The listing builds one solid part. Answer for the finished solid, in the listing's coordinates (mm). A direction names the side the tool comes from. Give positions to 0.01 mm unless a question says otherwise; leave off trailing zeros. Order: outer loops, then holes, each group sorted by start corner. A loop starts at its lowest first (then second) coordinate and runs counter-clockwise, first axis right, second up. Notation, with made-up numbers: (64, 59.25) - (120, 59.25) arc R15 ccw to (120, 77.25) - close; hole circle Ø11 at (34, -11). An arc over 180 degrees is marked (long way). Answer as CSV lines item,"result". Start each with the question number.
1. Section B-B on y = 21.5 is taken. Give the vertices of the cut face in (x, z) (3 decimals), and give its area (3 significant figures).
2. Section A-A on x = -26 is taken. Give the vertices of the cut face in (y, z) (3 decimals).
3. Consider line 1 along X through (y, z) = (4, 0.5); line 2 along X through (y, z) = (1.5, 2.75); line 3 along X through (y, z) = (22, 2.3). Determine where each line is inside the solid, lowest interval first. Write a range as [from, to].
4. Determine the mould class of faces 6 (the flat face through (-47, 79.301, 2)), 7 (the flat face through (-32.899, 4, 2)), 8 (the flat face through (-2, -3.884, 2)), 9 (the flat face through (50.286, 22, 2)) for opening direction X: +X half, -X half, draft (parallel to the pull), parting line (faces both ways), or undercut.
5. Which of the six approach directions +Z, -Z, +X, -X, +Y, -Y give full straight-line access (tool end or side, diameter ignored) to faces 1 (the flat face through (-32.899, -2, 2)), 2 (the flat face through (-1.307, 2, 2)), 3 (the flat face through (52, 26.926, 2)), 4 (the flat face through (-47, 1.831, 2)), 5 (the flat face through (-47, 45.493, 2))?
6. Flat-ended cylindrical pins translate along their axes: pin 1 (1 mm diameter, centred on x = -46, z = 1.5, fed in from -Y); pin 2 (1 mm diameter, centred on y = 44, z = 1, fed in from -X); pin 3 (1 mm diameter, centred on y = -6, z = 1, fed in from +X). Find the tip coordinate at first contact, or state that the pin passes through.
from build123d import *

# Parameters (mm, degrees)
F0_W     = 3.175
F0_H     = 6.35
F0_W_2   = 3.5052
F0_H_2   = 4.445
F0_H_3   = 2.778125
F0_W_3   = 2.21615
F0_H_4   = 2.301875
F1_DEPTH = 3.175


with BuildPart() as f1:
    # F0 (on Top) → F1 (new body)
    with BuildSketch(Plane.XY):
        with BuildLine():
            Line((-39.248683933, 94.5405161858), (-44.963683933, 94.5405161858))
            Line((-44.963683933, 94.5405161858), (-44.963683933, 85.6505161858))
            Line((-44.963683933, 85.6505161858), (-44.963683933, 79.3005161858))
            Line((-44.963683933, 79.3005161858), (-44.963683933, 75.7953161858))
            Line((-44.963683933, 75.7953161858), (-44.963683933, 69.4453161858))
            Line((-44.963683933, 69.4453161858), (-44.963683933, 51.8431161858))
            Line((-44.963683933, 51.8431161858), (-44.963683933, 45.4931161858))
            Line((-44.963683933, 45.4931161858), (-44.963683933, 43.7405161858))
            Line((-44.963683933, 43.7405161858), (50.286316067, 43.7405161858))
            Line((50.286316067, 43.7405161858), (50.286316067, 45.4931161858))
            Line((50.286316067, 45.4931161858), (50.286316067, 47.4018817204))
            ThreePointArc((50.286316067, 47.4018817204), (33.6573996556, 74.7365997743), (6.3226816016, 91.3655161858))
            Line((6.3226816016, 91.3655161858), (4.413916067, 91.3655161858))
            Line((4.413916067, 91.3655161858), (4.413916067, 86.9205161858))
            Line((4.413916067, 86.9205161858), (6.630066067, 86.9205161858))
            Line((6.630066067, 86.9205161858), (6.630066067, 84.1423911858))
            Line((6.630066067, 84.1423911858), (4.413916067, 84.1423911858))
            Line((4.413916067, 84.1423911858), (4.413916067, 81.8405161858))
            Line((4.413916067, 81.8405161858), (0.908716067, 81.8405161858))
            Line((0.908716067, 81.8405161858), (0.908716067, 84.1423911858))
            Line((0.908716067, 84.1423911858), (-1.307433933, 84.1423911858))
            Line((-1.307433933, 84.1423911858), (-1.307433933, 86.9205161858))
            Line((-1.307433933, 86.9205161858), (0.908716067, 86.9205161858))
            Line((0.908716067, 86.9205161858), (0.908716067, 91.3655161858))
            Line((0.908716067, 91.3655161858), (-5.441283933, 91.3655161858))
            Line((-5.441283933, 91.3655161858), (-5.441283933, 93.9768813524))
            ThreePointArc((-5.441283933, 93.9768813524), (-9.7882773782, 94.3994603443), (-14.153483933, 94.5405161858))
            Line((-14.153483933, 94.5405161858), (-23.043483933, 94.5405161858))
            Line((-23.043483933, 94.5405161858), (-23.043483933, 91.3655161858))
            Line((-23.043483933, 91.3655161858), (-29.393483933, 91.3655161858))
            Line((-29.393483933, 91.3655161858), (-29.393483933, 86.9205161858))
            Line((-29.393483933, 86.9205161858), (-27.177333933, 86.9205161858))
            Line((-27.177333933, 86.9205161858), (-27.177333933, 84.1423911858))
            Line((-27.177333933, 84.1423911858), (-29.393483933, 84.1423911858))
            Line((-29.393483933, 84.1423911858), (-29.393483933, 81.8405161858))
            Line((-29.393483933, 81.8405161858), (-32.898683933, 81.8405161858))
            Line((-32.898683933, 81.8405161858), (-32.898683933, 84.1423911858))
            Line((-32.898683933, 84.1423911858), (-35.114833933, 84.1423911858))
            Line((-35.114833933, 84.1423911858), (-35.114833933, 86.9205161858))
            Line((-35.114833933, 86.9205161858), (-32.898683933, 86.9205161858))
            Line((-32.898683933, 86.9205161858), (-32.898683933, 91.3655161858))
            Line((-32.898683933, 91.3655161858), (-39.248683933, 91.3655161858))
            Line((-39.248683933, 91.3655161858), (-39.248683933, 94.5405161858))
        make_face()
        with Locations((-46.551183933, 82.4755161858)):
            Rectangle(F0_W, F0_H)
        with Locations((-46.551183933, 72.6203161858)):
            Rectangle(F0_W, F0_H)
        with Locations((-46.551183933, 48.6681161858)):
            Rectangle(F0_W, F0_H)
        with BuildLine():
            ThreePointArc((0.908716067, 92.8415057221), (-2.252736339, 93.4849633701), (-5.441283933, 93.9768813524))
            Line((-5.441283933, 93.9768813524), (-5.441283933, 91.3655161858))
            Line((-5.441283933, 91.3655161858), (0.908716067, 91.3655161858))
            Line((0.908716067, 91.3655161858), (0.908716067, 92.8415057221))
        make_face()
        with BuildLine():
            ThreePointArc((4.413916067, 91.9411976981), (2.6673405912, 92.4148071961), (0.908716067, 92.8415057221))
            Line((0.908716067, 92.8415057221), (0.908716067, 91.3655161858))
            Line((0.908716067, 91.3655161858), (4.413916067, 91.3655161858))
            Line((4.413916067, 91.3655161858), (4.413916067, 91.9411976981))
        make_face()
        Polygon((50.286316067, 43.7405161858), (-44.963683933, 43.7405161858), (-44.963683933, 41.9879161858), (-44.963683933, 35.6379161858), (-44.963683933, 18.0357161858), (-44.963683933, 11.6857161858), (-44.963683933, 8.1805161858), (-44.963683933, 1.8305161858), (-44.963683933, -7.0594838142), (-39.248683933, -7.0594838142), (-39.248683933, -3.8844838142), (-32.898683933, -3.8844838142), (-32.898683933, 0.5605161858), (-35.114833933, 0.5605161858), (-35.114833933, 3.3386411858), (-32.898683933, 3.3386411858), (-32.898683933, 5.6405161858), (-29.393483933, 5.6405161858), (-29.393483933, 3.3386411858), (-27.177333933, 3.3386411858), (-27.177333933, 0.5605161858), (-29.393483933, 0.5605161858), (-29.393483933, -3.8844838142), (-23.043483933, -3.8844838142), (-23.043483933, -7.0594838142), (-5.441283933, -7.0594838142), (-5.441283933, -3.8844838142), (0.908716067, -3.8844838142), (0.908716067, 0.5605161858), (-1.307433933, 0.5605161858), (-1.307433933, 3.3386411858), (0.908716067, 3.3386411858), (0.908716067, 5.6405161858), (4.413916067, 5.6405161858), (4.413916067, 3.3386411858), (6.630066067, 3.3386411858), (6.630066067, 0.5605161858), (4.413916067, 0.5605161858), (4.413916067, -3.8844838142), (10.763916067, -3.8844838142), (10.763916067, -7.0594838142), (28.366116067, -7.0594838142), (28.366116067, -3.8844838142), (34.716116067, -3.8844838142), (34.716116067, 0.5605161858), (32.499966067, 0.5605161858), (32.499966067, 3.3386411858), (34.716116067, 3.3386411858), (34.716116067, 5.6405161858), (38.221316067, 5.6405161858), (38.221316067, 3.3386411858), (40.437466067, 3.3386411858), (40.437466067, 0.5605161858), (38.221316067, 0.5605161858), (38.221316067, -3.8844838142), (44.571316067, -3.8844838142), (44.571316067, -7.0594838142), (50.286316067, -7.0594838142), (50.286316067, 1.8305161858), (50.286316067, 8.1805161858), (50.286316067, 11.6857161858), (50.286316067, 18.0357161858), (50.286316067, 26.9257161858), (50.286316067, 35.6379161858), (50.286316067, 41.9879161858), align=None)
        with Locations((-46.551183933, 38.8129161858)):
            Rectangle(F0_W, F0_H)
        with Locations((2.661316067, 89.1430161858)):
            Rectangle(F0_W_2, F0_H_2)
        with BuildLine():
            ThreePointArc((6.3226816016, 91.3655161858), (5.3704207665, 91.6603925526), (4.413916067, 91.9411976981))
            Line((4.413916067, 91.9411976981), (4.413916067, 91.3655161858))
            Line((4.413916067, 91.3655161858), (6.3226816016, 91.3655161858))
        make_face()
        with BuildLine():
            Line((50.286316067, 45.4931161858), (50.286316067, 43.7405161858))
            Line((50.286316067, 43.7405161858), (51.3371541766, 43.7405161858))
            ThreePointArc((51.3371541766, 43.7405161858), (51.1054596409, 44.6184113637), (50.8619975793, 45.4931161858))
            Line((50.8619975793, 45.4931161858), (50.286316067, 45.4931161858))
        make_face()
        with BuildLine():
            Line((51.3371541766, 43.7405161858), (50.286316067, 43.7405161858))
            Line((50.286316067, 43.7405161858), (50.286316067, 41.9879161858))
            Line((50.286316067, 41.9879161858), (51.7623056033, 41.9879161858))
            ThreePointArc((51.7623056033, 41.9879161858), (51.5555733449, 42.8656337101), (51.3371541766, 43.7405161858))
        make_face()
        with Locations((2.661316067, 85.5314536858)):
            Rectangle(F0_W_2, F0_H_3)
        with Locations((-0.199358933, 85.5314536858)):
            Rectangle(F0_W_3, F0_H_3)
        with BuildLine():
            Line((51.7623056033, 41.9879161858), (50.286316067, 41.9879161858))
            Line((50.286316067, 41.9879161858), (50.286316067, 35.6379161858))
            Line((50.286316067, 35.6379161858), (52.8976812336, 35.6379161858))
            ThreePointArc((52.8976812336, 35.6379161858), (52.4057632513, 38.8264637797), (51.7623056033, 41.9879161858))
        make_face()
        with BuildLine():
            Line((50.286316067, 47.4018817204), (50.286316067, 45.4931161858))
            Line((50.286316067, 45.4931161858), (50.8619975793, 45.4931161858))
            ThreePointArc((50.8619975793, 45.4931161858), (50.5811924339, 46.4496208852), (50.286316067, 47.4018817204))
        make_face()
        with Locations((-46.551183933, 14.8607161858)):
            Rectangle(F0_W, F0_H)
        with Locations((5.521991067, 85.5314536858)):
            Rectangle(F0_W_3, F0_H_3)
        with Locations((2.661316067, 82.9914536858)):
            Rectangle(F0_W_2, F0_H_4)
        with BuildLine():
            Line((52.8976812336, 35.6379161858), (50.286316067, 35.6379161858))
            Line((50.286316067, 35.6379161858), (50.286316067, 26.9257161858))
            Line((50.286316067, 26.9257161858), (53.461316067, 26.9257161858))
            ThreePointArc((53.461316067, 26.9257161858), (53.3202602255, 31.2909227406), (52.8976812336, 35.6379161858))
        make_face()
        with Locations((-46.551183933, 5.0055161858)):
            Rectangle(F0_W, F0_H)
        with Locations((51.873816067, 14.8607161858)):
            Rectangle(F0_W, F0_H)
        with Locations((51.873816067, 5.0055161858)):
            Rectangle(F0_W, F0_H)
    extrude(amount=F1_DEPTH)


solid = f1.part
Checks:
1,outline,"(-44.964, 0) - (50.286, 0) - (50.286, 3.175) - (-44.964, 3.175) - close"
1,area,"302 mm²"
2,outline,"(-3.884, 0) - (91.366, 0) - (91.366, 3.175) - (-3.884, 3.175) - close"
3,line 1,"x = [-48.14, -32.9], [-29.39, 0.91], [4.41, 34.72], [38.22, 53.46]"
3,line 2,"x = [-44.96, -35.11], [-27.18, -1.31], [6.63, 32.5], [40.44, 50.29]"
3,line 3,"x = [-44.96, 50.29]"
4,face 6,"draft"
4,face 7,"undercut"
4,face 8,"undercut"
4,face 9,"+X half"
5,face 1,"+Z, -Z, -Y"
5,face 2,"+Z, -Z"
5,face 3,"+Z, -Z, +X"
5,face 4,"+Z, -Z, -X, -Y"
5,face 5,"+Z, -Z, -X"
6,pin 1,"stops at y = 1.83"
6,pin 2,"stops at x = -44.96"
6,pin 3,"stops at x = 50.29"
